Design review of the part built by this model. Coordinates are the model's own, in mm. A direction names the side the tool comes from. Round coordinates to 2 decimals unless told otherwise and drop trailing zeros. Order: outer loops, then holes, each group sorted by start corner. A loop starts at its lowest first (then second) coordinate and runs counter-clockwise, first axis right, second up. Notation, with made-up numbers: M 49.25,51 L 103.25,51 A27 ccw 103.25,75 Z; hole C 30,78.5 d9. An arc over 180 degrees is marked long. Write item = value, one per line. Start each with the question number.
```python
from build123d import *

# Parameters (mm, degrees)
F0_R     = 50
F1_DEPTH = 80
F2_R     = 100
F3_DEPTH = 5
F4_R     = 100
F5_DEPTH = 5
F6_R     = 27.5
F7_DEPTH = 100


with BuildPart() as f1:
    # F0 (on Front) → F1 (new body)
    with BuildSketch(Plane.XZ):
        Circle(F0_R)
    extrude(amount=F1_DEPTH)

    # F2 (on Front) → F3 (join)
    with BuildSketch(Plane.XZ):
        Circle(F2_R)
    extrude(amount=F3_DEPTH)

    # F4 (on face) → F5 (join)
    with BuildSketch(Plane.XZ.offset(80)):
        Circle(F4_R)
    extrude(amount=-F5_DEPTH)

    # F6 (on face) → F7 (cut)
    with BuildSketch(Plane(origin=(0, 0, 0), x_dir=(-1, 0, 0), z_dir=(0, 1, 0))):
        Circle(F6_R)
    extrude(amount=-F7_DEPTH, mode=Mode.SUBTRACT)


solid = f1.part
```
(1) Insertion check: pin 1 (3 mm diameter, centred on y = -36.5, z = -26, fed in from +X); pin 2 (10 mm diameter, centred on x = 15, y = -65.5, fed in from +Z); pin 3 (8 mm diameter, centred on y = -57.5, z = -8, fed in from -X). Each pin has a flat end and moves straight along its axis. Give the tip position at first contact, or say it passes through.
(2) Consider section C-C, the plane y = -70.5. Write out the cut boundary in (x, z), then the cut area to 3 significant figures.
(3) Consider section D-D, the plane x = 41.5. Write out the cut boundary in (y, z).
(4) Consider section A-A, the plane x = 0. Write out the cut boundary in (y, z).
(5) For faces 5 (the face through (5.961, -39.44, -26.846)), 6 (the face through (-46, -75, -21)), list the 3-axis set-ups (+Z, -Z, +X, -X, +Y, -Y) from which the entire face can be reached by the end or side of a thin tool; tool diameter is ignored.
(6) For line 1 along Y through (x, z) = (60, -53.5); line 2 along Z through (x, y) = (0, -30); line 3 along X through (y, z) = (-71, -1), list the stretches that pass through material, from the lowest coordinate up. Write a range as [from, to].
(7) Consider section B-B, the plane z = 0. Write out the cut boundary in (x, y).
(8) Draft analysis for pull direction Y (two halves, no side actions). For faces 1 (the face through (95.38, -77.54, 30.04)), 2 (the face through (-46, -5, -21)), 3 (the face through (21, -80, -21)), 4 (the face through (47.69, -39.51, 15.02)), state which applies: pulls with the +Y half, pulls with the -Y half, needs draft (parallel to the pull), parting line crosses it, or undercut.
Completed:
q1.pin_1 = 43.59
q1.pin_2 = 48.99
q1.pin_3 = -49.84
q2.outline = C 0,0 d100; hole C 0,0 d55
q2.area = 5,480 mm2
q3.outline = M -80,-90.98 L -75,-90.98 L -75,-27.89 L -5,-27.89 L -5,-90.98 L 0,-90.98 L 0,90.98 L -5,90.98 L -5,27.89 L -75,27.89 L -75,90.98 L -80,90.98 Z
q4.outline = M -80,-100 L -75,-100 L -75,-50 L -5,-50 L -5,-100 L 0,-100 L 0,-27.5 L -80,-27.5 Z; M -80,27.5 L 0,27.5 L 0,100 L -5,100 L -5,50 L -75,50 L -75,100 L -80,100 Z
q5.face_5 = +Y, -Y
q5.face_6 = none
q6.line_1 = [-80, -75], [-5, 0]
q6.line_2 = [-50, -27.5], [27.5, 50]
q6.line_3 = [-49.99, -27.48], [27.48, 49.99]
q7.outline = M -100,-80 L -27.5,-80 L -27.5,0 L -100,0 L -100,-5 L -50,-5 L -50,-75 L -100,-75 Z; M 27.5,-80 L 100,-80 L 100,-75 L 50,-75 L 50,-5 L 100,-5 L 100,0 L 27.5,0 Z
q8.face_1 = needs draft
q8.face_2 = undercut
q8.face_3 = pulls with the -Y half
q8.face_4 = undercut
